```python
from build123d import *

# Parameters (mm, degrees)
BOSS_EXTRUDE2_DEPTH = 10
SKETCH2_W           = 6
SKETCH2_H           = 21.5
CUT_EXTRUDE1_DEPTH  = 2
SKETCH18_W          = 10
SKETCH18_H          = 4
CUT_EXTRUDE6_DEPTH  = 2.32
BOSS_EXTRUDE4_DEPTH = 35.965
SKETCH20_W          = 10
SKETCH20_H          = 4.318
BOSS_EXTRUDE5_DEPTH = 9
SKETCH21_W          = 2
SKETCH21_H          = 57.465
BOSS_EXTRUDE6_DEPTH = 0.889
BOSS_EXTRUDE7_DEPTH = 9.02
CUT_EXTRUDE7_DEPTH  = 1.016
SKETCH24_W          = 4.069
SKETCH24_H          = 2.54
CUT_EXTRUDE8_DEPTH  = 1
SKETCH30_R          = 0.75565
CUT_EXTRUDE14_DEPTH = 95.738007626
SKETCH34_R          = 1.5
CUT_EXTRUDE18_DEPTH = 10
SKETCH35_R          = 0.75
CUT_EXTRUDE19_DEPTH = 60.59814159
SKETCH36_W          = 6
SKETCH36_H          = 10
CUT_EXTRUDE20_DEPTH = 10
SKETCH37_W          = 9
SKETCH37_H          = 2
BOSS_EXTRUDE8_DEPTH = 3.65
SKETCH38_W          = 4.069
SKETCH38_H          = 10
BOSS_EXTRUDE9_DEPTH = 3
SKETCH39_R          = 0.75
CUT_EXTRUDE21_DEPTH = 3
SKETCH40_W          = 0.381
SKETCH40_H          = 10
CUT_EXTRUDE22_DEPTH = 69.478136839


with BuildPart() as part:
    # Sketch1 → Boss-Extrude2 (new body)
    with BuildSketch(Plane.XY):
        Polygon((-4, 0), (-0.82, 0), (-0.82, 21.5), (-6.32, 21.5), (-6.32, 17.5), (-4, 17.5), align=None)
    extrude(amount=BOSS_EXTRUDE2_DEPTH)

    # Sketch2 → Cut-Extrude1 (cut)
    with BuildSketch(Plane(origin=(-0.82, 0, 0), x_dir=(0, 0, -1), z_dir=(1, 0, 0))):
        with Locations((-5, 10.75)):
            Rectangle(SKETCH2_W, SKETCH2_H)
    extrude(amount=-CUT_EXTRUDE1_DEPTH, mode=Mode.SUBTRACT)

    # Sketch18 → Cut-Extrude6 (cut)
    with BuildSketch(Plane.ZY.offset(6.32)):
        with Locations((5, 19.5)):
            Rectangle(SKETCH18_W, SKETCH18_H)
    extrude(amount=-CUT_EXTRUDE6_DEPTH, mode=Mode.SUBTRACT)

    # Sketch19 → Boss-Extrude4 (add)
    with BuildSketch(Plane(origin=(0, 21.5, 0), x_dir=(1, 0, 0), z_dir=(0, 1, 0))):
        Polygon((-0.82, -10), (-4, -10), (-4, 0), (-0.82, 0), (-0.82, -2), (-2.82, -2), (-2.82, -8), (-0.82, -8), align=None)
    extrude(amount=BOSS_EXTRUDE4_DEPTH)

    # Sketch20 → Boss-Extrude5 (add)
    with BuildSketch(Plane.ZY.offset(4)):
        with Locations((5, 55.306)):
            Rectangle(SKETCH20_W, SKETCH20_H)
    extrude(amount=BOSS_EXTRUDE5_DEPTH)

    # Sketch21 → Boss-Extrude6 (add)
    with BuildSketch(Plane(origin=(-0.82, 0, 0), x_dir=(0, 0, -1), z_dir=(1, 0, 0))):
        with Locations((-9, 28.7325)):
            Rectangle(SKETCH21_W, SKETCH21_H)
        with Locations((-1, 28.7325)):
            Rectangle(SKETCH21_W, SKETCH21_H)
    extrude(amount=BOSS_EXTRUDE6_DEPTH)

    # Sketch22 → Boss-Extrude7 (add)
    with BuildSketch(Plane.XZ):
        Polygon((-4, 10), (0.069, 10), (0.069, 8), (-2.82, 8), (-2.82, 2), (0.069, 2), (0.069, 0), (-4, 0), align=None)
    extrude(amount=BOSS_EXTRUDE7_DEPTH)

    # Sketch23 → Cut-Extrude7 (cut)
    with BuildSketch(Plane.XY.offset(10)):
        Polygon((0.069, -3.02), (0.069, -4.29), (-4, -4.29), (-4, -1.75), (0.069, -1.75), align=None)
        Polygon((-4, 47.426731456), (-4, 48.696731456), (0.069, 48.696731456), (0.069, 46.156731456), (-4, 46.156731456), align=None)
    extrude(amount=-CUT_EXTRUDE7_DEPTH, mode=Mode.SUBTRACT)

    # Sketch24 → Cut-Extrude8 (cut)
    with BuildSketch(Plane.XY.offset(10)):
        with Locations((-1.9655, 35.355048592)):
            Rectangle(SKETCH24_W, SKETCH24_H)
    extrude(amount=-CUT_EXTRUDE8_DEPTH, mode=Mode.SUBTRACT)

    # Sketch30 → Cut-Extrude14 (cut, through all)
    with BuildSketch(Plane(origin=(35.063086629, -23.678267082, 9), x_dir=(1, 0, 0), z_dir=(0, 0, 1))):
        with Locations((-36.581586629, 59.033315674)):
            Circle(SKETCH30_R)
    extrude(amount=-CUT_EXTRUDE14_DEPTH, mode=Mode.SUBTRACT)

    # Sketch34 → Cut-Extrude18 (cut)
    with BuildSketch(Plane(origin=(0, 57.465, 0), x_dir=(1, 0, 0), z_dir=(0, 1, 0))):
        with Locations(Location((-9.5, -5, 0), (0, 0, 270))):
            Circle(SKETCH34_R)
    extrude(amount=-CUT_EXTRUDE18_DEPTH, mode=Mode.SUBTRACT)

    # Sketch35 → Cut-Extrude19 (cut, through all)
    with BuildSketch(Plane.XY.offset(8.984)):
        with Locations((-1.5185, 47.456731456)):
            Circle(SKETCH35_R)
        with Locations((-1.5185, -3.05)):
            Circle(SKETCH35_R)
    extrude(amount=-CUT_EXTRUDE19_DEPTH, mode=Mode.SUBTRACT)

    # Sketch36 → Cut-Extrude20 (cut)
    with BuildSketch(Plane(origin=(-2.82, 0, 0), x_dir=(0, 0, -1), z_dir=(1, 0, 0))):
        with Locations((-5, 48.147)):
            Rectangle(SKETCH36_W, SKETCH36_H)
    extrude(amount=-CUT_EXTRUDE20_DEPTH, mode=Mode.SUBTRACT)

    # Sketch37 → Boss-Extrude8 (add)
    with BuildSketch(Plane.XZ.offset(-53.147)):
        with Locations((-8.5, 9)):
            Rectangle(SKETCH37_W, SKETCH37_H)
        with Locations((-8.5, 1)):
            Rectangle(SKETCH37_W, SKETCH37_H)
    extrude(amount=BOSS_EXTRUDE8_DEPTH)

    # Sketch38 → Boss-Extrude9 (add)
    with BuildSketch(Plane.XZ.offset(9.02)):
        with Locations((-1.9655, 5)):
            Rectangle(SKETCH38_W, SKETCH38_H)
    extrude(amount=-BOSS_EXTRUDE9_DEPTH)

    # Sketch39 → Cut-Extrude21 (cut)
    with BuildSketch(Plane.XZ.offset(9.02)):
        with Locations(Location((-1.7, 5, 0), (0, 0, 270))):
            Circle(SKETCH39_R)
    extrude(amount=-CUT_EXTRUDE21_DEPTH, mode=Mode.SUBTRACT)

    # Sketch40 → Cut-Extrude22 (cut, through all)
    with BuildSketch(Plane(origin=(0, 57.465, 0), x_dir=(1, 0, 0), z_dir=(0, 1, 0))):
        with Locations((-0.1215, -5)):
            Rectangle(SKETCH40_W, SKETCH40_H)
    extrude(amount=-CUT_EXTRUDE22_DEPTH, mode=Mode.SUBTRACT)


solid = part.part
```
Geometry check sheet. Reference: the model listing, model coordinates, mm. A direction names the side the tool comes from. Give positions to 0.01 mm unless a question says otherwise; leave off trailing zeros. Loops run counter-clockwise (first coordinate to the right, second up) from the corner with the lowest first, then second, coordinate; pieces in that order, holes last. Notation, with made-up numbers: M -28.75,64 L 28.25,64 A8 ccw 28.25,79 Z; hole C 56,42 d10. An arc over 180 degrees is marked long. Write item = value, one per line. Start each with the question number.
1. Tool access check on faces 5 (the face through (-9, 49.497, 9)), 6 (the face through (-1, -6.02, 6)), 7 (the face through (-7.8, 53.147, 5)). Record the directions out of +Z, -Z, +X, -X, +Y, -Y that give a thin tool (end or side, any length) a straight path to the whole face; none if there is none.
2. Section check B-B, the plane y = -3.05. Enter the section's corners in (x, z).
3. Section check C-C, the plane x = -7.25. Enter the section's corners in (y, z) (3 decimals).
4. Section check D-D, the plane y = 33.5. Enter the section's corners in (x, z).
5. Go/stop test with flat-tipped pins: P1, Ø0.8, axis at x = -2.5, y = -3.5, coming from the +Z side; P2, Ø2.5, axis at x = -9.5, z = 5, coming from the -Y side; P3, Ø2, axis at x = -9.5, z = 1, coming from the -Y side; P4, Ø1, axis at x = -5.5, z = 5, coming from the -Y side. Record where each tip stops, or that it passes through.
6. Draft check along Z on faces 1 (the face through (-3, 43.147, 5)), 2 (the face through (-7, 53, 10)), 3 (the face through (-9, 49.497, 1)), 4 (the face through (-3.7, 32.1, 0)). Enter one of: +Z half, -Z half, draft (parallel to the pull), parting line (faces both ways), or undercut.
7. Thickness scan on probe 1 along X at (y, z) = (54.3, 5); probe 2 along Z at (x, y) = (-2.5, -5.5); probe 3 along Z at (x, y) = (-3.25, 48). Record the ranges inside material, lowest first.
8. Section check A-A, the plane z = 5. Enter the section's corners in (x, y) (3 decimals).
Values follow:
q1.face_5 = +Z, -Z, -X, -Y
q1.face_6 = +X, +Y
q1.face_7 = +X, -X
q2.outline = M -4,0 L -2.27,0 L -2.27,2 L -2.82,2 L -2.82,8 L -2.27,8 L -2.27,8.98 L -4,8.98 Z; M -0.77,0 L -0.31,0 L -0.31,2 L -0.77,2 Z; M -0.77,8 L -0.31,8 L -0.31,8.98 L -0.77,8.98 Z
q3.outline = M 49.497,0 L 57.465,0 L 57.465,10 L 49.497,10 L 49.497,8 L 53.147,8 L 53.147,2 L 49.497,2 Z
q4.outline = M -4,0 L -0.31,0 L -0.31,2 L -2.82,2 L -2.82,8 L -0.31,8 L -0.31,10 L -4,10 Z
q5.P1 = 8.98
q5.P2 = through
q5.P3 = 49.5
q5.P4 = 53.15
q6.face_1 = undercut
q6.face_2 = +Z half
q6.face_3 = draft
q6.face_4 = -Z half
q7.probe_1 = -13 to -11, -8 to -2.82
q7.probe_2 = 0 to 2, 8 to 10
q7.probe_3 = 0 to 2, 8 to 8.98
q8.outline = M -13,53.147 L -11,53.147 L -11,57.465 L -13,57.465 Z; M -8,53.147 L -2.82,53.147 L -2.82,57.465 L -8,57.465 Z; M -4,-9.02 L -2.45,-9.02 L -2.45,-6.02 L -2.82,-6.02 L -2.82,43.147 L -4,43.147 Z; M -0.95,-9.02 L -0.312,-9.02 L -0.312,-6.02 L -0.95,-6.02 Z
